Here's how the part is built. I have some questions about the finished solid (model axes, mm). A direction names the side the tool comes from. Give positions to 0.01 mm unless a question says otherwise; leave off trailing zeros. Loops run counter-clockwise (first coordinate to the right, second up) from the corner with the lowest first, then second, coordinate; pieces in that order, holes last.
Q1. Suppose I cut it at A-A (z = -3.75). Count the separate pieces of the cut face and the enclosed holes in it, and give its area (3 significant figures).
Q2. For faces 4 (the face through (171, 88.595, -3)), 5 (the face through (172.7, 71, -3)), 6 (the face through (-9, 101.595, -3)), which set-ups out of +Z, -Z, +X, -X, +Y, -Y let a thin tool reach every point of the face, with its end or its side?
Q3. I'm going to push flat-ended pins straight in: P1, Ø1.1, axis at y = 54, z = -4.5, coming from the -X side; P2, Ø3.5, axis at y = 52, z = -2.5, coming from the +X side. Where does each tip first touch, or does it pass through?
Q4. I need wall thicknesses on probe 1 along Y at (x, z) = (131.15, -2.5); probe 2 along X at (y, z) = (87.5, -3.3); probe 3 along X at (y, z) = (81, -0.45). Which ranges of each line are inside material? Lowest first, please.
Q5. Thinking about a two-plate mould opening in Y: for faces 1 (the face through (172.7, 100, -3)), 2 (the face through (82, 107.595, -3)), 3 (the face through (40.317, 42.902, -3.042)), which applies, pulls with the +Y half, pulls with the -Y half, needs draft (parallel to the pull), parting line crosses it, or undercut?
Q6. Suppose I cut it at B-B (y = 47). List the corners of the cut face in (x, z) for me, and give its area (3 significant figures).
```python
from build123d import *

# Parameters (mm, degrees)
SZKIC1_W                    = 178.7
SZKIC1_H                    = 69
DODANIE_WYCI_GNI_CIE1_DEPTH = 6
SZKIC3_R                    = 1.55
WYTNIJ_WYCI_GNI_CIE1_DEPTH  = 204.563124249
WYTNIJ_WYCI_GNI_CIE2_DEPTH  = 204.563124249
SZYK_LINIOWY1_COUNT         = 2
SZYK_LINIOWY1_PITCH         = 38
SZKIC5_W                    = 6
SZKIC5_H                    = 6
DODANIE_WYCI_GNI_CIE2_DEPTH = 5.8


with BuildPart() as part:
    # Szkic1 → Dodanie-wyciągnięcie1 (new body)
    with BuildSketch(Plane.XY):
        with Locations((83.35, 73.094867693)):
            Rectangle(SZKIC1_W, SZKIC1_H)
    extrude(amount=-DODANIE_WYCI_GNI_CIE1_DEPTH)

    # Szkic3 → Wytnij-wyciągnięcie1 (cut, through all)
    with BuildSketch(Plane(origin=(0, 0, -6), x_dir=(-1, 0, 0), z_dir=(0, 0, -1))):
        with Locations((-41.15, 41.594867693)):
            Circle(SZKIC3_R)
        with Locations((-131.15, 41.594867693)):
            Circle(SZKIC3_R)
    extrude(amount=-WYTNIJ_WYCI_GNI_CIE1_DEPTH, mode=Mode.SUBTRACT)

    # Szkic4 → Wytnij-wyciągnięcie2 (cut, through all)
    with BuildSketch(Plane(origin=(0, 0, -6), x_dir=(-1, 0, 0), z_dir=(0, 0, -1))):
        Polygon((-172.7, 50.594867693), (-172.7, 53.694867693), (-168.7, 53.694867693), (-168.7, 55.069867693), (-166.7, 55.069867693), (-166.7, 53.694867693), (-166.2, 53.694867693), (-166.2, 50.594867693), (-166.7, 50.594867693), (-166.7, 49.219867693), (-168.7, 49.219867693), (-168.7, 50.594867693), align=None)
    wytnij_wyci_gni_cie2 = extrude(amount=-WYTNIJ_WYCI_GNI_CIE2_DEPTH, mode=Mode.SUBTRACT)

    # Szyk liniowy1: Wytnij-wyciągnięcie2 ×2
    with Locations(*[(0, i * SZYK_LINIOWY1_PITCH, 0) for i in range(1, SZYK_LINIOWY1_COUNT)]):
        add(wytnij_wyci_gni_cie2, mode=Mode.SUBTRACT)

    # Szkic5 → Dodanie-wyciągnięcie2 (add)
    with BuildSketch(Plane.ZY.offset(6)):
        with Locations((-3, 104.594867693)):
            Rectangle(SZKIC5_W, SZKIC5_H)
    extrude(amount=DODANIE_WYCI_GNI_CIE2_DEPTH)


solid = part.part
```
Solutions:
1. separate pieces: 1
1. enclosed holes: 2
1. area: 12,300 mm2
2. face 4: +Z, -Z, +X
2. face 5: +Z, -Z, +X, +Y, -Y
2. face 6: +Z, -Z, -X, -Y
3. P1: stops at x = -6
3. P2: stops at x = 172.7
4. probe 1: y = 38.59 to 40.04, 43.14 to 107.59
4. probe 2: x = -6 to 166.7, 168.7 to 172.7
4. probe 3: x = -6 to 172.7
5. face 1: needs draft
5. face 2: pulls with the +Y half
5. face 3: undercut
6. outline: (-6, -6) - (172.7, -6) - (172.7, 0) - (-6, 0) - close
6. area: 1,070 mm2
